Could you check a few things on this model? Use its own coordinates, in mm. A direction names the side the tool comes from. Coordinates: 2 decimals unless noted, no trailing zeros. Order: outer loops, then holes, each group sorted by start corner. A loop starts at its lowest first (then second) coordinate and runs counter-clockwise, first axis right, second up. Notation, with made-up numbers: (55.25, 8) -> (110.25, 8) arc R13 cw to (110.25, 25) -> close; hole circle Ø9 at (75.25, 79). An arc over 180 degrees is marked (long way). Use a Markdown table: item, result. Add a question column.
1) If I drill on L1, parallel to Z at x = -7.5, y = 2.25; L2, parallel to Z at x = 0, y = 1.4; L3, parallel to Z at x = -7.5, y = 4.3, over which ranges is the centre line in solid material (lowest first)? Write a range as [from, to].
2) Thinking about a two-plate mould opening in Z: for faces 3 (the flat face through (-17, 2, 0)), 4 (the cylindrical face through (-7.77, 1.52, 14.21)), 5 (the cylindrical face through (19.987, 2.465, -0.724)), which applies, +Z half, -Z half, draft (parallel to the pull), parting line (faces both ways), or undercut?
3) If we section it at B-B (z = 0): Write out the boundary of the cut face in (x, y).
4) If we section it at D-D (z = 5): Write out the boundary of the cut face in (x, y), plus the area to 3 significant figures.
5) If we section it at C-C (x = -7.5): Write out the boundary of the cut face in (y, z), plus the area to 3 significant figures.
6) If we section it at A-A (x = 0): Write out the boundary of the cut face in (y, z), plus the area to 4 significant figures.
7) Will these pins go through, and if not, where does the flat tip stop? pin 1 Ø3 at (x, y) = (-3.5, 4) entering from -Z; pin 2 Ø2 at (x, y) = (-12, 4) entering from -Z; pin 3 Ø1.5 at (x, z) = (-8.5, -12) entering from +Y.
8) Which directions (+Z, -Z, +X, -X, +Y, -Y) give clear straight access to the entire face, cutting with the end or side of a thin tool? Please do faces 1 (the cylindrical face through (13.75, 1.52, -0.05)), 2 (the cylindrical face through (-6.32, 4.01, -10.73)).
Autodesk Inventor part; units mm, degrees
ref_plane "YZ Plane" through (0, 0, 0) normal (1, 0, 0) x (0, 1, 0)
ref_plane "XZ Plane" through (0, 0, 0) normal (0, 1, 0) x (-1, 0, 0)
ref_plane "XY Plane" through (0, 0, 0) normal (0, 0, 1) x (1, 0, 0)
sketch "Sketch1" plane through (0, 0, 0) normal (0, 1, 0) x (-1, 0, 0)
  circle A0 centre (0, 0) radius 8.75
  circle A1 centre (0, 0) radius 20
  dimension "d0" = 17.5
  dimension "d1" = 40
extrude "Extrusion1" add sketch "Sketch1" along normal blind 5
sketch "Sketch2" plane through (0, 5, 0) normal (0, 1, 0) x (1, 0, 0)
  circle A0 centre (0, 0) radius 15 construction
  circle A1 centre (15, 0) radius 2.55
  circle A2 centre (0, 0) radius 15 construction
  circle A3 centre (-7.5, 12.9904) radius 2.55
  circle A4 centre (0, 0) radius 15 construction
  circle A5 centre (-7.5, -12.9904) radius 2.55
  dimension "d4" = 30
  dimension "d5" = 5.1
  dimension "d8" = 360
extrude "Extrusion3" cut sketch "Sketch2" against normal blind 2
sketch "Sketch3" plane through (-7.5, 3, 12.9904) normal (0, 1, 0) x (1, 0, 0)
  circle A0 centre (0, 0) radius 1.25
  circle A1 centre (22.5, 12.9904) radius 2.55
  circle A2 centre (22.5, 12.9904) radius 1.25
  circle A3 centre (0, 25.9808) radius 2.55
  circle A4 centre (0, 25.9808) radius 1.25
  point P0 (7.5, 12.9904)
  dimension "d14" = 2.5
  dimension "d15" = 2.5
  dimension "d16" = 2.5
extrude "Extrusion4" cut sketch "Sketch3" against normal blind 3 contours A0 | A2 | A4
sketch "Sketch4" plane through (0, 0, 0) normal (0, -1, 0) x (1, 0, 0)
  line L0 (-17, -45) -> (-17, 22)
  arc A0 (-17, 10.5357) -> (-17, -10.5357) centre (0, 0) ccw
extrude "Extrusion5" cut sketch "Sketch4" against normal blind 10
properties part number "modified_o_ring"
Answer sheet:
| question | item | result |
|---|---|---|
| 1 | L1 | [-18.54, -14.24], [-11.74, -4.51], [4.51, 11.74], [14.24, 18.54] |
| 1 | L2 | [-20, -8.75], [8.75, 20] |
| 1 | L3 | [-18.54, -15.54], [-10.44, -4.51], [4.51, 10.44], [15.54, 18.54] |
| 2 | face 3 | draft |
| 2 | face 4 | undercut |
| 2 | face 5 | parting line |
| 3 | outline | (-17, 0) -> (-8.75, 0) -> (-8.75, 5) -> (-17, 5) -> close; (8.75, 0) -> (13.75, 0) -> (13.75, 3) -> (12.45, 3) -> (12.45, 5) -> (8.75, 5) -> close; (16.25, 0) -> (20, 0) -> (20, 5) -> (17.55, 5) -> (17.55, 3) -> (16.25, 3) -> close |
| 4 | outline | (-17, 0) -> (-7.18, 0) -> (-7.18, 5) -> (-17, 5) -> close; (7.18, 0) -> (19.36, 0) -> (19.36, 5) -> (7.18, 5) -> close |
| 4 | area | 110 mm2 |
| 5 | outline | (0, -18.54) -> (5, -18.54) -> (5, -15.54) -> (3, -15.54) -> (3, -14.24) -> (0, -14.24) -> close; (0, -11.74) -> (3, -11.74) -> (3, -10.44) -> (5, -10.44) -> (5, -4.51) -> (0, -4.51) -> close; (0, 4.51) -> (5, 4.51) -> (5, 10.44) -> (3, 10.44) -> (3, 11.74) -> (0, 11.74) -> close; (0, 14.24) -> (3, 14.24) -> (3, 15.54) -> (5, 15.54) -> (5, 18.54) -> (0, 18.54) -> close |
| 5 | area | 105 mm2 |
| 6 | outline | (0, -20) -> (5, -20) -> (5, -8.75) -> (0, -8.75) -> close; (0, 8.75) -> (5, 8.75) -> (5, 20) -> (0, 20) -> close |
| 6 | area | 112.5 mm2 |
| 7 | pin 1 | z = -19.9 |
| 7 | pin 2 | z = -16.7 |
| 7 | pin 3 | y = 3 |
| 8 | face 1 | +Y, -Y |
| 8 | face 2 | +Y |
